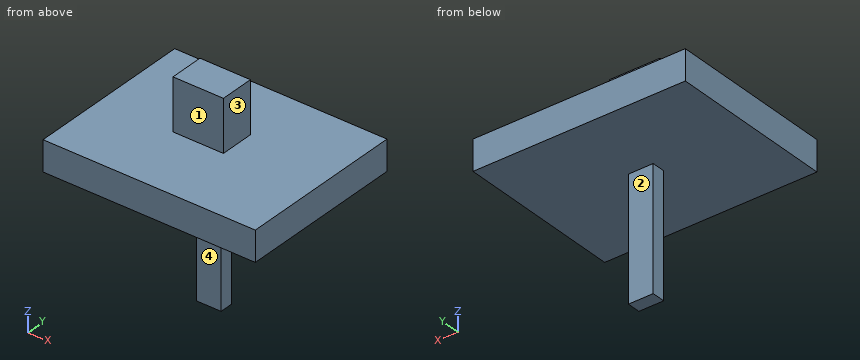
```python
from build123d import *

# Parameters (mm, degrees)
F0_W     = 10.811692
F0_H     = 66.33117
F1_DEPTH = 5.8
F2_W     = 92.621132
F2_H     = 73.195636
F2_W_2   = 10.811692
F2_H_2   = 5.8
F3_DEPTH = 13.2
F4_W     = 22
F4_H     = 15
F5_DEPTH = 22.5


with BuildPart() as f1:
    # F0 (on Front) → F1 (new body)
    with BuildSketch(Plane.XZ):
        Rectangle(F0_W, F0_H)
    extrude(amount=F1_DEPTH)

    # F2 (on face) → F3 (join)
    with BuildSketch(Plane.XY.offset(33.165585)):
        with Locations((0, -2.3061)):
            Rectangle(F2_W, F2_H)
        with Locations((0, -2.9)):
            Rectangle(F2_W_2, F2_H_2, mode=Mode.SUBTRACT)
    extrude(amount=-F3_DEPTH)

    # F4 (on face) → F5 (join)
    with BuildSketch(Plane.XY.offset(33.165585)):
        with Locations((-3.245262, 0)):
            Rectangle(F4_W, F4_H)
    extrude(amount=F5_DEPTH)


solid = f1.part
```
Model file for the job. Use its own axes, mm. Face numbers are marked on the shaded views. A direction names the side the tool comes from. Coordinates: 2 decimals unless noted, no trailing zeros. Order: outer loops, then holes, each group sorted by start corner. A loop starts at its lowest first (then second) coordinate and runs counter-clockwise, first axis right, second up. Notation, with made-up numbers: (-38, 85) - (-12, 85) arc R21 ccw to (-12, 108) - close; hole circle Ø6 at (46.5, 31.5). An arc over 180 degrees is marked (long way). Return JSON: item names as keys, results as strings. Group by question number.
1) Saw through at C-C, the plane x = -27.5. Write the cut outline in (y, z).
2) Saw through at B-B, the plane z = 49. Write the cut outline in (x, y).
3) Saw through at A-A, the plane y = -3. Write the cut outline in (x, z).
4) Flat gauge pins, fed straight in: P1, Ø8, axis at x = 20.5, z = 39.5, coming from the +Y side; P2, Ø3, axis at y = -3, z = -2, coming from the +X side; P3, Ø16.5, axis at y = 0, z = 43, coming from the +X side; P4, Ø3, axis at x = -18.5, y = 8, coming from the +Z side. Where does each tip first touch, or does it go through?
5) Probe line 1 (Z direction, x = 40, y = -12.5); line 2 (Y direction, x = -0.5, z = 18.5); line 3 (X direction, y = -4.5, z = -10.5). List the from-to ranges inside material, lowest first. Write a range as from..to.
6) Tool access for the marked faces 1, 2, 3 and 4: list every direction of +Z, -Z, +X, -X, +Y, -Y with a clear straight run to the whole face (end or side of a thin tool).
Values found:
{
 "1": {"outline": "(-38.9, 19.97) - (34.29, 19.97) - (34.29, 33.17) - (-38.9, 33.17) - close"},
 "2": {"outline": "(-14.25, -7.5) - (7.75, -7.5) - (7.75, 7.5) - (-14.25, 7.5) - close"},
 "3": {"outline": "(-46.31, 19.97) - (-5.41, 19.97) - (-5.41, -33.17) - (5.41, -33.17) - (5.41, 19.97) - (46.31, 19.97) - (46.31, 33.17) - (7.75, 33.17) - (7.75, 55.67) - (-14.25, 55.67) - (-14.25, 33.17) - (-46.31, 33.17) - close"},
 "4": {"P1": "passes through", "P2": "stops at x = 5.41", "P3": "stops at x = 7.75", "P4": "stops at z = 33.17"},
 "5": {"line 1": "z = 19.97..33.17", "line 2": "y = -5.8..0", "line 3": "x = -5.41..5.41"},
 "6": {"face 1": "+Z, +X, -X, -Y", "face 2": "-Z, +X, -X, +Y", "face 3": "+Z, +X, +Y, -Y", "face 4": "-Z, +X, -X, -Y"}
}
